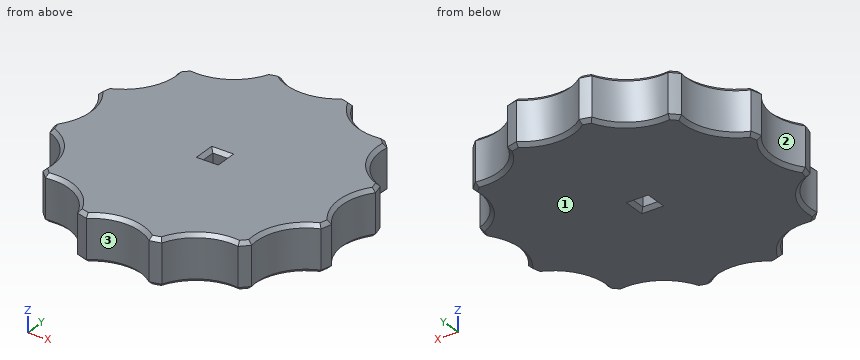
```python
from build123d import *

# Parameters (mm, degrees)
SKIZZE1_R                       = 20
SKIZZE1_W                       = 2.08
SKIZZE1_H                       = 2.08
AUFSATZ_LINEAR_AUSTRAGEN1_DEPTH = 6.5
SCHNITT_LINEAR_AUSTRAGEN1_DEPTH = 6.5
KREISMUSTER1_COUNT              = 12
FASE1_SIZE                      = 0.5


with BuildPart() as part:
    # Skizze1 → Aufsatz-Linear austragen1 (new body)
    with BuildSketch(Plane.XY):
        with Locations(Location((0, 0, 0), (0, 0, 180))):
            Circle(SKIZZE1_R)
        Rectangle(SKIZZE1_W, SKIZZE1_H, mode=Mode.SUBTRACT)
    extrude(amount=AUFSATZ_LINEAR_AUSTRAGEN1_DEPTH)

    # Skizze2 → Schnitt-Linear austragen1 (cut)
    with BuildSketch(Plane.XY):
        with BuildLine():
            Line((-5.535516041, 20.658827109), (5.535516041, 20.658827109))
            ThreePointArc((5.535516041, 20.658827109), (0, 17.943458035), (-5.535516041, 20.658827109))
        make_face()
    schnitt_linear_austragen1 = extrude(amount=SCHNITT_LINEAR_AUSTRAGEN1_DEPTH, mode=Mode.SUBTRACT)

    # Kreismuster1: Schnitt-Linear austragen1 ×12 about axis
    kreismuster1_axis = Axis((0, 0, 0), (0, 0, 1))
    for i in range(1, KREISMUSTER1_COUNT):
        add(schnitt_linear_austragen1.rotate(kreismuster1_axis, i * 360 / KREISMUSTER1_COUNT), mode=Mode.SUBTRACT)

    # Fase1
    fase1_edges = [part.edges().sort_by_distance(p)[0] for p in [
        (1.04, 0, 6.5),
        (0, 1.04, 6.5),
        (-19.318516526, 5.176380902, 0),
        (-15.53949049, 8.971729017, 0),
        (-19.318516526, 5.176380902, 6.5),
        (-15.53949049, 8.971729017, 6.5),
        (-14.142135624, -14.142135624, 0),
        (-15.53949049, -8.971729017, 0),
        (-14.142135624, -14.142135624, 6.5),
        (-15.53949049, -8.971729017, 6.5),
        (5.176380902, -19.318516526, 0),
        (0, -17.943458035, 0),
        (5.176380902, -19.318516526, 6.5),
        (0, -17.943458035, 6.5),
        (19.318516526, -5.176380902, 0),
        (15.53949049, -8.971729017, 0),
        (19.318516526, -5.176380902, 6.5),
        (15.53949049, -8.971729017, 6.5),
        (14.142135624, 14.142135624, 0),
        (15.53949049, 8.971729017, 0),
        (14.142135624, 14.142135624, 6.5),
        (15.53949049, 8.971729017, 6.5),
        (-5.176380902, 19.318516526, 6.5),
        (-5.176380902, 19.318516526, 0),
        (0, 17.943458035, 0),
        (0, 17.943458035, 6.5),
        (-14.142135624, 14.142135624, 0),
        (-19.318516526, -5.176380902, 0),
        (-5.176380902, -19.318516526, 0),
        (14.142135624, -14.142135624, 0),
        (19.318516526, 5.176380902, 0),
        (5.176380902, 19.318516526, 0),
        (-8.971729017, 15.53949049, 0),
        (-17.943458035, 0, 0),
        (-8.971729017, -15.53949049, 0),
        (8.971729017, -15.53949049, 0),
        (17.943458035, 0, 0),
        (8.971729017, 15.53949049, 0),
        (-14.142135624, 14.142135624, 6.5),
        (-19.318516526, -5.176380902, 6.5),
        (-5.176380902, -19.318516526, 6.5),
        (14.142135624, -14.142135624, 6.5),
        (19.318516526, 5.176380902, 6.5),
        (5.176380902, 19.318516526, 6.5),
        (8.971729017, 15.53949049, 6.5),
        (17.943458035, 0, 6.5),
        (8.971729017, -15.53949049, 6.5),
        (-8.971729017, -15.53949049, 6.5),
        (-1.04, 0, 0),
        (0, -1.04, 0),
        (-17.943458035, 0, 6.5),
        (1.04, 0, 0),
        (-8.971729017, 15.53949049, 6.5),
        (0, 1.04, 0),
        (-1.04, 0, 6.5),
        (0, -1.04, 6.5),
    ]]
    chamfer(fase1_edges, length=FASE1_SIZE)


solid = part.part
```
Here's how the part is built. I have some questions about the finished solid (model axes, mm). Face numbers are marked on the shaded views. Coordinates: 2 decimals unless noted, no trailing zeros. Loops run counter-clockwise (first coordinate to the right, second up) from the corner with the lowest first, then second, coordinate; pieces in that order, holes last. Notation, with made-up numbers: M 76.25,0.5 L 87.25,0.5 A20 ccw 87.25,14.5 Z; hole C 42.25,59 d1. An arc over 180 degrees is marked long. One line per item, written item: value.
1. Will these pins go through, and if not, where does the flat tip stop? pin 1 Ø3 at (x, z) = (-12.5, 1) entering from +Y; pin 2 Ø1.5 at (y, z) = (2.5, 4.5) entering from +X; pin 3 Ø1.7 at (y, z) = (-0.5, 3.5) entering from -X.
Geometry says:
pin 1: stops at y = 14.76
pin 2: stops at x = 18.74
pin 3: stops at x = -18.07
2. Thinking about a two-plate mould opening in X: for the marked faces 1, 2 and 3, which applies, +X half, -X half, draft (parallel to the pull), parting line (faces both ways), or undercut?
Geometry says:
face 1: draft
face 2: -X half
face 3: undercut
3. Please list where these lines run through material, in increasing order: probe 1 along Y at (x, z) = (6.5, 2.5); probe 2 along Y at (x, z) = (-12.5, 2.25); probe 3 along X at (y, z) = (0.5, 3.75).
Geometry says:
probe 1: y = -17.95 to 17.95
probe 2: y = -14.6 to 14.6
probe 3: x = -17.96 to -1.04, 1.04 to 17.96
4. Imagine slicing it at A-A (z = 5.25). List the corners of the cut face in (x, y) for me.
Geometry says:
outline: M -19.51,-4.41 A20 ccw -19.1,-5.93 A7 cw -14.69,-13.57 A20 ccw -13.57,-14.69 A7 cw -5.93,-19.1 A20 ccw -4.41,-19.51 A7 cw 4.41,-19.51 A20 ccw 5.93,-19.1 A7 cw 13.57,-14.69 A20 ccw 14.69,-13.57 A7 cw 19.1,-5.93 A20 ccw 19.51,-4.41 A7 cw 19.51,4.41 A20 ccw 19.1,5.93 A7 cw 14.69,13.57 A20 ccw 13.57,14.69 A7 cw 5.93,19.1 A20 ccw 4.41,19.51 A7 cw -4.41,19.51 A20 ccw -5.93,19.1 A7 cw -13.57,14.69 A20 ccw -14.69,13.57 A7 cw -19.1,5.93 A20 ccw -19.51,4.41 A7 cw Z; hole M -1.04,-1.04 L 1.04,-1.04 L 1.04,1.04 L -1.04,1.04 Z
